Design review of the part built by this model. Coordinates are the model's own, in mm. Round coordinates to 2 decimals unless told otherwise and drop trailing zeros. Loops run counter-clockwise (first coordinate to the right, second up) from the corner with the lowest first, then second, coordinate; pieces in that order, holes last. Notation, with made-up numbers: M -23.75,67 L 0.25,67 A26 cw 0.25,100 Z; hole C 1,-24.75 d9. An arc over 180 degrees is marked long. One line per item, written item: value. Start each with the question number.
Item 1: We need section A-A (y = 0). Write out the cut boundary in (x, z) (3 decimals), then the cut area to 3 significant figures.
Item 2: We need section C-C (z = 79.5). Write out the cut boundary in (x, y) (3 decimals).
Item 3: For line 1 along Y through (x, z) = (7.62, 20) (3 decimals); line 2 along X through (y, z) = (12.7, 26.5) (3 decimals); line 3 along X through (y, z) = (0.5, 6), list the stretches that pass through material, from the lowest coordinate up.
Item 4: We need section D-D (y = 28). Write out the cut boundary in (x, z).
Item 5: Clearance check with flat-ended pins moving along their axes: pin 1 (12 mm diameter, centred on x = -44.5, y = 19, fed in from -Z); pin 2 (1.5 mm diameter, centred on x = -16.5, z = 53.5, fed in from +Y); pin 3 (3 mm diameter, centred on x = 30, z = 66, fed in from +Y); pin 4 (4 mm diameter, centred on x = 59.5, y = 32.5, fed in from +Z). State where each tip first meets the part, or that it passes through.
Item 6: We need section B-B (x = -7.62). Write out the cut boundary in (y, z) (3 decimals).
from build123d import *

# Parameters (mm, degrees)
F0_W     = 152.4
F0_H     = 101.6
F1_DEPTH = 34.29
F5_D     = 6.35


with BuildPart() as f1:
    # F0 (on Top) → F1 (new body)
    with BuildSketch(Plane.XY):
        Rectangle(F0_W, F0_H)
    extrude(amount=F1_DEPTH)

    # F2 (on Front) → F3 (revolve)
    with BuildSketch(Plane.XZ):
        with BuildLine():
            Line((0, 88.9), (0, 0))
            ThreePointArc((0, 0), (44.45, 44.45), (0, 88.9))
        make_face()
    revolve(axis=Axis((0, 0, 44.45), (0, 0, 1)))

    # F5 (through all)
    with Locations(Plane(origin=(0, 0, 0), x_dir=(1, 0, 0), z_dir=(0, 0, -1))):
        with Locations((-7.62, 12.7), (7.62, 12.7), (-7.62, 0), (7.62, -12.7), (-7.62, -12.7), (7.62, 0)):
            Hole(F5_D / 2)


solid = f1.part
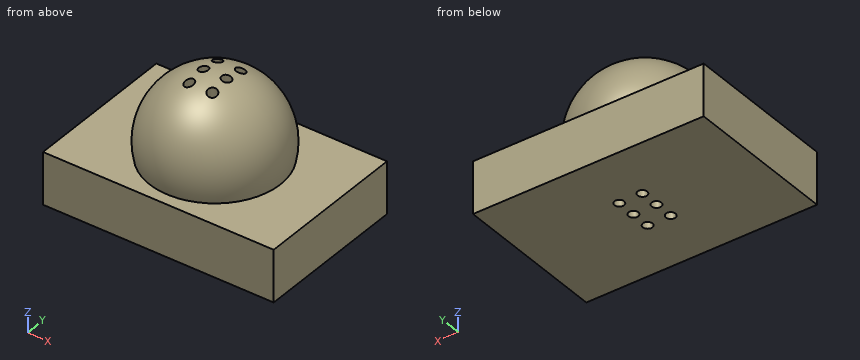
A:
1. outline: M -76.2,0 L -10.795,0 L -10.795,87.569 A44.45 ccw -43.273,34.29 L -76.2,34.29 Z; M -4.445,0 L 4.445,0 L 4.445,88.677 A44.45 ccw -4.445,88.677 Z; M 10.795,0 L 76.2,0 L 76.2,34.29 L 43.273,34.29 A44.45 ccw 10.795,87.569 Z
1. area: 8,100 mm2
2. outline: C 0,0 d54.674; hole C -7.62,-12.7 d6.35; hole C -7.62,0 d6.35; hole C -7.62,12.7 d6.35; hole C 7.62,-12.7 d6.35; hole C 7.62,0 d6.35; hole C 7.62,12.7 d6.35
3. line 1: -50.8 to -15.875, -9.525 to -3.175, 3.175 to 9.525, 15.875 to 50.8
3. line 2: -76.2 to -10.795, -4.445 to 4.445, 10.795 to 76.2
3. line 3: -76.2 to -10.76, -4.48 to 4.48, 10.76 to 76.2
4. outline: M -76.2,0 L 76.2,0 L 76.2,34.29 L 32.99,34.29 A34.52 ccw long -32.99,34.29 L -76.2,34.29 Z
5. pin 1: z = 0
5. pin 2: y = 40.61
5. pin 3: y = 26.83
5. pin 4: z = 34.29
6. outline: M -50.8,0 L -15.875,0 L -15.875,85.263 A43.792 ccw -42.597,34.29 L -50.8,34.29 Z; M -9.525,0 L -3.175,0 L -3.175,88.127 A43.792 ccw -9.525,87.194 Z; M 3.175,0 L 9.525,0 L 9.525,87.194 A43.792 ccw 3.175,88.127 Z; M 15.875,0 L 50.8,0 L 50.8,34.29 L 42.597,34.29 A43.792 ccw 15.875,85.263 Z
